Source: CAD feature listing. Evaluate the final solid. Frame: model axes, mm. Face numbers are marked on the shaded views. A direction names the side the tool comes from. Give positions to 0.01 mm unless a question says otherwise; leave off trailing zeros. Loops run counter-clockwise (first coordinate to the right, second up) from the corner with the lowest first, then second, coordinate; pieces in that order, holes last. Notation, with made-up numbers: M 54.5,71 L 67.5,71 A18 ccw 67.5,96 Z; hole C 37,44.25 d1. An arc over 180 degrees is marked long. Put each result on its own line as item: value.
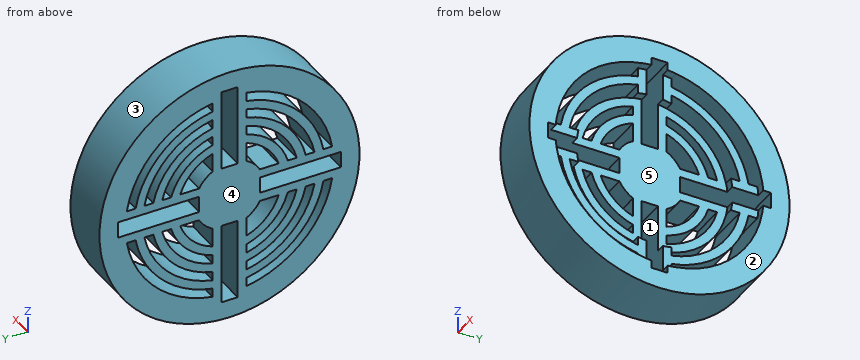
from build123d import *

# Parameters (mm, degrees)
BOSS_EXTRUDE1_OUTLINE_R   = 7.5
BOSS_EXTRUDE1_OUTLINE_W   = 0.935836939
BOSS_EXTRUDE1_OUTLINE_H   = 4.677443156
BOSS_EXTRUDE1_OUTLINE_W_2 = 4.677419546
BOSS_EXTRUDE1_OUTLINE_H_2 = 0.93583693
BOSS_EXTRUDE1_DEPTH       = 3
CUT_EXTRUDE1_START        = -0.5
SKETCH2_R                 = 6
CUT_EXTRUDE1_DEPTH        = 0.5
CUT_EXTRUDE2_START        = -0.5
SKETCH3_R                 = 4.5
CUT_EXTRUDE2_DEPTH        = 0.5


# Read off the part's stored shape, not the designer's step: Boss-Extrude1
with BuildPart() as part:
    # Boss-Extrude1 outline → Boss-Extrude1 (new body)
    with BuildSketch(Plane(origin=(0, 0, 0), x_dir=(0, 0, -1), z_dir=(1, 0, 0))):
        Circle(BOSS_EXTRUDE1_OUTLINE_R)
        with Locations((-5e-09, -4.088902667)):
            Rectangle(BOSS_EXTRUDE1_OUTLINE_W, BOSS_EXTRUDE1_OUTLINE_H, mode=Mode.SUBTRACT)
        with BuildLine():
            ThreePointArc((-5.414160493, -0.967918465), (-3.889087297, -3.889087297), (-0.967918465, -5.414160493))
            Line((-0.967918465, -5.414160493), (-0.967918465, -5.921413163))
            ThreePointArc((-0.967918465, -5.921413163), (-4.242640687, -4.242640687), (-5.921413163, -0.967918465))
            Line((-5.921413163, -0.967918465), (-5.414160493, -0.967918465))
        make_face(mode=Mode.SUBTRACT)
        with BuildLine():
            ThreePointArc((-4.394671074, -0.967918465), (-3.181980515, -3.181980515), (-0.967918465, -4.394671074))
            Line((-0.967918465, -4.394671074), (-0.967918465, -4.905418825))
            ThreePointArc((-0.967918465, -4.905418825), (-3.535533906, -3.535533906), (-4.905418825, -0.967918465))
            Line((-4.905418825, -0.967918465), (-4.394671074, -0.967918465))
        make_face(mode=Mode.SUBTRACT)
        with BuildLine():
            ThreePointArc((-3.363500237, -0.967918465), (-2.474873734, -2.474873734), (-0.967918465, -3.363500237))
            Line((-0.967918465, -3.363500237), (-0.967918465, -3.881125332))
            ThreePointArc((-0.967918465, -3.881125332), (-2.828427125, -2.828427125), (-3.881125332, -0.967918465))
            Line((-3.881125332, -0.967918465), (-3.363500237, -0.967918465))
        make_face(mode=Mode.SUBTRACT)
        with BuildLine():
            ThreePointArc((-1.750181089, -0.967918465), (-1.414213562, -1.414213562), (-0.967918465, -1.750181089))
            Line((-0.967918465, -1.750181089), (-0.967918465, -2.839565785))
            ThreePointArc((-0.967918465, -2.839565785), (-2.121320344, -2.121320344), (-2.839565785, -0.967918465))
            Line((-2.839565785, -0.967918465), (-1.750181089, -0.967918465))
        make_face(mode=Mode.SUBTRACT)
        with BuildLine():
            Line((5.414160493, -0.967918465), (5.921413163, -0.967918465))
            ThreePointArc((5.921413163, -0.967918465), (4.242640687, -4.242640687), (0.967918465, -5.921413163))
            Line((0.967918465, -5.921413163), (0.967918465, -5.414160493))
            ThreePointArc((0.967918465, -5.414160493), (3.889087297, -3.889087297), (5.414160493, -0.967918465))
        make_face(mode=Mode.SUBTRACT)
        with BuildLine():
            Line((4.394671074, -0.967918465), (4.905418825, -0.967918465))
            ThreePointArc((4.905418825, -0.967918465), (3.535533906, -3.535533906), (0.967918465, -4.905418825))
            Line((0.967918465, -4.905418825), (0.967918465, -4.394671074))
            ThreePointArc((0.967918465, -4.394671074), (3.181980515, -3.181980515), (4.394671074, -0.967918465))
        make_face(mode=Mode.SUBTRACT)
        with BuildLine():
            Line((3.363500237, -0.967918465), (3.881125332, -0.967918465))
            ThreePointArc((3.881125332, -0.967918465), (2.828427125, -2.828427125), (0.967918465, -3.881125332))
            Line((0.967918465, -3.881125332), (0.967918465, -3.363500237))
            ThreePointArc((0.967918465, -3.363500237), (2.474873734, -2.474873734), (3.363500237, -0.967918465))
        make_face(mode=Mode.SUBTRACT)
        with BuildLine():
            Line((1.750181089, -0.967918465), (2.839565785, -0.967918465))
            ThreePointArc((2.839565785, -0.967918465), (2.121320344, -2.121320344), (0.967918465, -2.839565785))
            Line((0.967918465, -2.839565785), (0.967918465, -1.750181089))
            ThreePointArc((0.967918465, -1.750181089), (1.414213562, -1.414213562), (1.750181089, -0.967918465))
        make_face(mode=Mode.SUBTRACT)
        with Locations((-4.088890862, 0)):
            Rectangle(BOSS_EXTRUDE1_OUTLINE_W_2, BOSS_EXTRUDE1_OUTLINE_H_2, mode=Mode.SUBTRACT)
        with BuildLine():
            ThreePointArc((-2.839565785, 0.967918465), (-2.121320344, 2.121320344), (-0.967918465, 2.839565785))
            Line((-0.967918465, 2.839565785), (-0.967918465, 1.750181089))
            ThreePointArc((-0.967918465, 1.750181089), (-1.414213562, 1.414213562), (-1.750181089, 0.967918465))
            Line((-1.750181089, 0.967918465), (-2.839565785, 0.967918465))
        make_face(mode=Mode.SUBTRACT)
        with BuildLine():
            Line((-3.363500237, 0.967918465), (-3.881125332, 0.967918465))
            ThreePointArc((-3.881125332, 0.967918465), (-2.828427125, 2.828427125), (-0.967918465, 3.881125332))
            Line((-0.967918465, 3.881125332), (-0.967918465, 3.363500237))
            ThreePointArc((-0.967918465, 3.363500237), (-2.474873734, 2.474873734), (-3.363500237, 0.967918465))
        make_face(mode=Mode.SUBTRACT)
        with BuildLine():
            ThreePointArc((-4.905418825, 0.967918465), (-3.535533906, 3.535533906), (-0.967918465, 4.905418825))
            Line((-0.967918465, 4.905418825), (-0.967918465, 4.394671074))
            ThreePointArc((-0.967918465, 4.394671074), (-3.181980515, 3.181980515), (-4.394671074, 0.967918465))
            Line((-4.394671074, 0.967918465), (-4.905418825, 0.967918465))
        make_face(mode=Mode.SUBTRACT)
        with BuildLine():
            ThreePointArc((-5.921413163, 0.967918465), (-4.242640687, 4.242640687), (-0.967918465, 5.921413163))
            Line((-0.967918465, 5.921413163), (-0.967918465, 5.414160493))
            ThreePointArc((-0.967918465, 5.414160493), (-3.889087297, 3.889087297), (-5.414160493, 0.967918465))
            Line((-5.414160493, 0.967918465), (-5.921413163, 0.967918465))
        make_face(mode=Mode.SUBTRACT)
        with Locations((-5e-09, 4.088902667)):
            Rectangle(BOSS_EXTRUDE1_OUTLINE_W, BOSS_EXTRUDE1_OUTLINE_H, mode=Mode.SUBTRACT)
        with BuildLine():
            Line((0.967918465, 1.750181089), (0.967918465, 2.839565785))
            ThreePointArc((0.967918465, 2.839565785), (2.121320344, 2.121320344), (2.839565785, 0.967918465))
            Line((2.839565785, 0.967918465), (1.750181089, 0.967918465))
            ThreePointArc((1.750181089, 0.967918465), (1.414213562, 1.414213562), (0.967918465, 1.750181089))
        make_face(mode=Mode.SUBTRACT)
        with BuildLine():
            Line((0.967918465, 3.363500237), (0.967918465, 3.881125332))
            ThreePointArc((0.967918465, 3.881125332), (2.828427125, 2.828427125), (3.881125332, 0.967918465))
            Line((3.881125332, 0.967918465), (3.363500237, 0.967918465))
            ThreePointArc((3.363500237, 0.967918465), (2.474873734, 2.474873734), (0.967918465, 3.363500237))
        make_face(mode=Mode.SUBTRACT)
        with BuildLine():
            Line((0.967918465, 4.394671074), (0.967918465, 4.905418825))
            ThreePointArc((0.967918465, 4.905418825), (3.535533906, 3.535533906), (4.905418825, 0.967918465))
            Line((4.905418825, 0.967918465), (4.394671074, 0.967918465))
            ThreePointArc((4.394671074, 0.967918465), (3.181980515, 3.181980515), (0.967918465, 4.394671074))
        make_face(mode=Mode.SUBTRACT)
        with BuildLine():
            Line((0.967918465, 5.414160493), (0.967918465, 5.921413163))
            ThreePointArc((0.967918465, 5.921413163), (4.242640687, 4.242640687), (5.921413163, 0.967918465))
            Line((5.921413163, 0.967918465), (5.414160493, 0.967918465))
            ThreePointArc((5.414160493, 0.967918465), (3.889087297, 3.889087297), (0.967918465, 5.414160493))
        make_face(mode=Mode.SUBTRACT)
        with Locations((4.088890862, 0)):
            Rectangle(BOSS_EXTRUDE1_OUTLINE_W_2, BOSS_EXTRUDE1_OUTLINE_H_2, mode=Mode.SUBTRACT)
    extrude(amount=BOSS_EXTRUDE1_DEPTH)

    # Sketch2 → Cut-Extrude1 (cut)
    with BuildSketch(Plane(origin=(3, 0, 0), x_dir=(0, 0, -1), z_dir=(1, 0, 0)).offset(CUT_EXTRUDE1_START)):
        Circle(SKETCH2_R)
    extrude(amount=CUT_EXTRUDE1_DEPTH, mode=Mode.SUBTRACT)

    # Sketch3 → Cut-Extrude2 (cut)
    with BuildSketch(Plane(origin=(2.5, 0, 0), x_dir=(0, 0, -1), z_dir=(1, 0, 0)).offset(CUT_EXTRUDE2_START)):
        Circle(SKETCH3_R)
    extrude(amount=CUT_EXTRUDE2_DEPTH, mode=Mode.SUBTRACT)


solid = part.part
1. Material intervals for line 1 (Y direction, x = 2.4, z = -0.25); line 2 (Y direction, x = 0.65, z = 4.5); line 3 (Z direction, x = 2.7, y = -5.25), sorted ascending. Write a range as from..to.
Found:
line 1: -7.5..-6.43, 6.43..7.5
line 2: -6..-3.97, -3.16..-2.18, -0.97..-0.47, 0.47..0.97, 2.18..3.16, 3.97..6
line 3: -5.36..-2.9, 2.9..5.36
2. Access query for the marked faces 1 and 2. Directions: +Z, -Z, +X, -X, +Y, -Y. A direction counts if a zero-diameter tool reaches every point of the face in a straight line with its end or side. Return the directions, or none.
Found:
face 1: +X, -X
face 2: +Z, -Z, +X, +Y, -Y
3. Section query C-C (x = 0.75). State how many separate pieces and enclosed holes the cut face has, plus the area to 3 significant figures.
Found:
separate pieces: 1
enclosed holes: 20
area: 118 mm^2
4. Draft query along Z for the marked faces 3, 4 and 5. Return one class per face: pulls with the +Z half, pulls with the -Z half, needs draft (parallel to the pull), parting line crosses it, or undercut.
Found:
face 3: parting line crosses it
face 4: needs draft
face 5: undercut
5. Section query A-A (y = 0). Output: boundary loops of the cut face in (x, z).
Found:
outline: M 0,-7.5 L 3,-7.5 L 3,-6.43 L 0,-6.43 Z; M 0,-1.75 L 2,-1.75 L 2,1.75 L 0,1.75 Z; M 0,6.43 L 3,6.43 L 3,7.5 L 0,7.5 Z
6. Contact query for flat-ended pins moving along their axis: P1, Ø0.9, axis at x = 2, y = 3, coming from the -Z side; P2, Ø6, axis at y = 2, z = 2, coming from the -X side; P3, Ø0.6, axis at x = 0.5, z = -3.5, coming from the +Y side; P4, Ø0.5, axis at x = 1, y = 2.5, coming from the +Z side. Output: stop coordinate, or through.
Found:
P1: z = -7.05
P2: x = 0
P3: y = 6.78
P4: z = 7.15
